Could you check a few things on this model? Use its own coordinates, in mm. A direction names the side the tool comes from. Coordinates: 2 decimals unless noted, no trailing zeros. Order: outer loops, then holes, each group sorted by start corner. A loop starts at its lowest first (then second) coordinate and runs counter-clockwise, first axis right, second up. Notation, with made-up numbers: (61.5, 56.5) -> (109.5, 56.5) arc R6 cw to (109.5, 61.5) -> close; hole circle Ø9 at (39.25, 85). An arc over 180 degrees is marked (long way). Put each result on its own line as item: value. Start each with the question number.
Q1. Please list where these lines run through material, in increasing order: line 1 along X through (y, z) = (4, 34); line 2 along X through (y, z) = (5.25, -11.5); line 3 along Z through (x, y) = (-10.5, 6.45).
Q2. For faces 1 (the face through (0, 7, -5.5)), 2 (the face through (-24.5, 0, -38.4)), 3 (the face through (21.488, 3, 37)), which set-ups out of +Z, -Z, +X, -X, +Y, -Y let a thin tool reach every point of the face, with its end or its side?
Q3. We'd pull the mould along X, two halves only. Please class faces 4 (the face through (5.5, 7, 0)), 5 (the face through (10, 9, -1)), 6 (the face through (44.734, 4.437, -14.087)): +X half, -X half, draft (parallel to the pull), parting line (faces both ways), or undercut.
Q4. If we section it at A-A (z = 0): Please give me the cut outline in (x, y), and give its area (3 significant figures).
Q5. Will these pins go through, and if not, where does the flat tip stop? pin 1 (3 mm diameter, centred on x = 0.5, y = 6.5, fed in from -Z); pin 2 (4.5 mm diameter, centred on x = -0.5, y = 8, fed in from +Z); pin 3 (2.5 mm diameter, centred on x = 41.05, z = -11, fed in from -Y).
from build123d import *

# Parameters (mm, degrees)
SKETCH_1_R          = 46.9
SKETCH_1_R_2        = 45.1
EXTRUDE_2_DEPTH     = 5
SKETCH_2_R          = 46.9
EXTRUDE_1_DEPTH     = 4
SKETCH_4_W          = 11
SKETCH_4_H          = 11
CUT_EXTRUDE_1_DEPTH = 67.514810381
HOLE_WIZARD_2_D     = 1.7
HOLE_WIZARD_2_DEPTH = 4.4
CHAMFER_1_SIZE      = 0.3
HOLE_WIZARD_1_D     = 1.7
EXTRUDE_2_2_DEPTH   = 4


with BuildPart() as part:
    # 草图1 → Extrude 2 (new body)
    with BuildSketch(Plane(origin=(0, 0, 0), x_dir=(1, 0, 0), z_dir=(0, 1, 0))):
        Circle(SKETCH_1_R)
        Circle(SKETCH_1_R_2, mode=Mode.SUBTRACT)
    extrude(amount=EXTRUDE_2_DEPTH)

    # 草图2 → 凸台-拉伸1 (add)
    with BuildSketch(Plane(origin=(0, 5, 0), x_dir=(1, 0, 0), z_dir=(0, 1, 0))):
        Circle(SKETCH_2_R)
    extrude(amount=EXTRUDE_1_DEPTH)

    # 草图4 → 切除-拉伸1 (cut, through all)
    with BuildSketch(Plane.XZ.offset(-5)):
        Rectangle(SKETCH_4_W, SKETCH_4_H)
    extrude(amount=-CUT_EXTRUDE_1_DEPTH, mode=Mode.SUBTRACT)

    # 孔2
    with Locations(Plane(origin=(0, 5, 0), x_dir=(-1, 0, 0), z_dir=(0, -1, 0))):
        with Locations((-1, 10.326086957), (10.5, 10.326086957), (10.5, -10.326086957), (-1, -10.326086957)):
            Hole(HOLE_WIZARD_2_D / 2, depth=HOLE_WIZARD_2_DEPTH)

    # 倒角1
    chamfer_1_edges = [part.edges().sort_by_distance(p)[0] for p in [
        (-45.1, 0, 0),
    ]]
    chamfer(chamfer_1_edges, length=CHAMFER_1_SIZE)

    # 孔1 (through all)
    with Locations(Plane(origin=(0, 9, 0), x_dir=(1, 0, 0), z_dir=(0, 1, 0))):
        with Locations((-41.051847617, 10.999809417), (-30.0520382, 30.0520382), (30.0520382, 30.0520382), (41.051847617, 10.999809417), (10.999809417, -41.051847617), (-10.999809417, -41.051847617)):
            Hole(HOLE_WIZARD_1_D / 2)

    # 草图20 → Extrude 2 2 (add)
    with BuildSketch(Plane.XZ.offset(-5)):
        with BuildLine():
            Line((17.668302266, 41.386363636), (17.668302266, 35.886363636))
            ThreePointArc((17.668302266, 35.886363636), (19.60780664, 34.86450801), (21.488415705, 33.737931034))
            Line((21.488415705, 33.737931034), (21.488415705, 39.537931034))
            ThreePointArc((21.488415705, 39.537931034), (19.60016113, 40.50720533), (17.668302266, 41.386363636))
        make_face()
    extrude(amount=EXTRUDE_2_2_DEPTH)


solid = part.part
The answers:
1. line 1: -32.3 to -29.63, 21.07 to 21.49, 29.63 to 32.3
1. line 2: -45.47 to -41.74, -40.36 to 40.36, 41.74 to 45.47
1. line 3: -45.71 to -11.18, -9.48 to 9.48, 11.18 to 40.36, 41.74 to 45.71
2. face 1: +Y, -Y
2. face 2: +Z, -Z, +X, -X, -Y
2. face 3: -Y
3. face 4: undercut
3. face 5: draft
3. face 6: parting line
4. outline: (-46.9, 0) -> (-45.4, 0) -> (-45.1, 0.3) -> (-45.1, 5) -> (-5.5, 5) -> (-5.5, 9) -> (-46.9, 9) -> close; (5.5, 5) -> (45.1, 5) -> (45.1, 0.3) -> (45.4, 0) -> (46.9, 0) -> (46.9, 9) -> (5.5, 9) -> close
4. area: 349 mm^2
5. pin 1: z = -46.9
5. pin 2: z = 46.9
5. pin 3: y = 5
